Work out the finished part from the listing and answer in its coordinate system (mm). A direction names the side the tool comes from. Round coordinates to 2 decimals unless told otherwise and drop trailing zeros. Loops run counter-clockwise (first coordinate to the right, second up) from the corner with the lowest first, then second, coordinate; pieces in that order, holes last. Notation, with made-up numbers: (-39.5, -27.75) - (-7.5, -27.75) arc R15 ccw to (-7.5, -13.75) - close; hole circle Ø3 at (-40, 68.5). An arc over 180 degrees is marked (long way). Use CSV: the item, a comma, the result in double quotes. Start each with the question number.
from build123d import *

# Parameters (mm, degrees)
F2_DEPTH  = 30
F1_R      = 32.262952
F1_R_2    = 24.574153
F4_DEPTH  = 55
F6_W      = 65.900745
F6_H      = 33.107504
F7_DEPTH  = 55
F8_W      = 65.835031
F8_H      = 35.700139
F9_DEPTH  = 55
F10_R     = 12.5
F11_DEPTH = 100
F12_R     = 12.5
F13_DEPTH = 100


with BuildPart() as f2:
    # F1 (on face) → F2 (new body)
    with BuildSketch(Plane.XZ):
        with BuildLine():
            Line((68.240136, 49.884874), (28.858346, 49.884874))
            ThreePointArc((28.858346, 49.884874), (-3.404606, 17.621922), (-35.667558, 49.884874))
            Line((-35.667558, 49.884874), (-67.648031, 49.884874))
            Line((-67.648031, 49.884874), (-67.648031, -49.884874))
            Line((-67.648031, -49.884874), (68.240136, -49.884874))
            Line((68.240136, -49.884874), (68.240136, 49.884874))
        make_face()
    extrude(amount=F2_DEPTH)

    # F3: F2 across face


with BuildPart() as f2_1:
    add(f2.part)
    add(f2.part.mirror(Plane(origin=(0.803557, 0, -4.963344), x_dir=(1, 0, 0), z_dir=(0, 1, 0))))

    # F1 (on face) → F4 (join)
    with BuildSketch(Plane.XZ):
        with Locations((-3.404606, 49.884874)):
            Circle(F1_R)
        with Locations((-3.404606, 49.884874)):
            Circle(F1_R_2, mode=Mode.SUBTRACT)
    extrude(amount=F4_DEPTH)

    # F5: F2 across face


with BuildPart() as f2_2:
    add(f2_1.part)
    add(f2_1.part.mirror(Plane(origin=(-3.404606, 0, 49.884874), x_dir=(1, 0, 0), z_dir=(0, 1, 0))))

    # F6 (on Front) → F7 (cut)
    with BuildSketch(Plane.XZ):
        with Locations((-2.747394, 66.43793)):
            Rectangle(F6_W, F6_H)
    extrude(amount=-F7_DEPTH, mode=Mode.SUBTRACT)

    # F8 (on Front) → F9 (cut)
    with BuildSketch(Plane.XZ):
        with Locations((-3.836475, 67.761236)):
            Rectangle(F8_W, F8_H)
    extrude(amount=F9_DEPTH, mode=Mode.SUBTRACT)

    # F10 (on face) → F11 (cut)
    with BuildSketch(Plane.XY.offset(49.884874)):
        with Locations((-50.148031, 0)):
            Circle(F10_R)
    extrude(amount=-F11_DEPTH, mode=Mode.SUBTRACT)

    # F12 (on face) → F13 (cut)
    with BuildSketch(Plane.XY.offset(49.884874)):
        with Locations((50.740136, 0)):
            Circle(F12_R)
    extrude(amount=-F13_DEPTH, mode=Mode.SUBTRACT)


solid = f2_2.part
Item 1: A cutting plane is placed at D-D (x = 6). Determine the outline of the cut face in (y, z), plus the area to 3 significant figures.
Item 2: Which of the six approach directions +Z, -Z, +X, -X, +Y, -Y give full straight-line access (tool end or side, diameter ignored) to faces 4 (the flat face through (68.24, 0, -1)), 5 (the cylindrical face through (-4.11, 42.32, 17.63))?
Item 3: A cutting plane is placed at C-C (y = -4). State how many separate pieces and enclosed holes the cut face has, plus the area to 3 significant figures.
Item 4: Each of these flat-tipped pins is pushed along its axis until it touches: pin 1 Ø12 at (x, z) = (-3, -14) entering from -Y; pin 2 Ø3 at (x, y) = (47.5, 11.5) entering from +Z; pin 3 Ø15 at (x, y) = (-50.15, 0) entering from -Z; pin 4 Ø3 at (x, z) = (40, -24) entering from +Y. Where does it stop, or does it pass through?
Item 5: A cutting plane is placed at B-B (z = -40). Determine the outline of the cut face in (x, y).
Item 6: Find the intervals of material crossed by probe 1 along Y at (x, z) = (15, -4.5); probe 2 along X at (y, z) = (2, -31); probe 3 along Z at (x, y) = (-57.5, 21.5), in increasing order. Write a range as [from, to].
Item 7: The mould has two halves that part along Y. Classify faces 1 (the cylindrical face through (-38.225, 3.755, 0.698)), 2 (the flat face through (-1, -30, 1)), 3 (the flat face through (-1, 0, -49.885)): pulls with the +Y half, pulls with the -Y half, needs draft (parallel to the pull), parting line crosses it, or undercut.
Result sheet:
1,outline,"(-55, 19.02) - (-30, 19.02) - (-30, -49.88) - (30, -49.88) - (30, 19.02) - (55, 19.02) - (55, 27.18) - (-55, 27.18) - close"
1,area,"5,030 mm^2"
2,face 4,"+Z, -Z, +X, +Y, -Y"
2,face 5,"-Z, +Y"
3,separate pieces,"3"
3,enclosed holes,"0"
3,area,"7,880 mm^2"
4,pin 1,"y = -30"
4,pin 2,"z = 49.88"
4,pin 3,"through"
4,pin 4,"y = 30"
5,outline,"(-67.65, -30) - (68.24, -30) - (68.24, 30) - (-67.65, 30) - close; hole circle Ø25 at (-50.15, 0); hole circle Ø25 at (50.74, 0)"
6,probe 1,"[-30, 30]"
6,probe 2,"[-67.65, -62.49], [-37.81, 38.4], [63.08, 68.24]"
6,probe 3,"[-49.88, 49.88]"
7,face 1,"undercut"
7,face 2,"pulls with the -Y half"
7,face 3,"needs draft"
